from build123d import *

# Parameters (mm, degrees)
SKETCH1_R           = 57.15
SKETCH1_R_2         = 1.397
SKETCH1_R_3         = 3.175
BOSS_EXTRUDE1_DEPTH = 4.572
SKETCH2_R           = 2.75
SKETCH2_R_2         = 1.75
BOSS_EXTRUDE2_DEPTH = 2
SKETCH3_R           = 5
SKETCH3_R_2         = 1.75
BOSS_EXTRUDE3_DEPTH = 3


with BuildPart() as part:
    # Sketch1 → Boss-Extrude1 (new body)
    with BuildSketch(Plane(origin=(0, 0, 0), x_dir=(1, 0, 0), z_dir=(0, 1, 0))):
        Circle(SKETCH1_R)
        with Locations((0, 6.35)):
            Circle(SKETCH1_R_2, mode=Mode.SUBTRACT)
        with Locations((0, 25.4)):
            Circle(SKETCH1_R_3, mode=Mode.SUBTRACT)
        with Locations((0, 50.8)):
            Circle(SKETCH1_R_3, mode=Mode.SUBTRACT)
        with Locations((25.4, 0)):
            Circle(SKETCH1_R_3, mode=Mode.SUBTRACT)
        with Locations((0, -25.4)):
            Circle(SKETCH1_R_3, mode=Mode.SUBTRACT)
        with Locations((-25.4, 0)):
            Circle(SKETCH1_R_3, mode=Mode.SUBTRACT)
        with Locations((6.35, 0)):
            Circle(SKETCH1_R_2, mode=Mode.SUBTRACT)
        with Locations((0, -6.35)):
            Circle(SKETCH1_R_2, mode=Mode.SUBTRACT)
        with Locations((-6.35, 0)):
            Circle(SKETCH1_R_2, mode=Mode.SUBTRACT)
        with Locations((35.921024484, 35.921024484)):
            Circle(SKETCH1_R_3, mode=Mode.SUBTRACT)
        with Locations((50.8, 0)):
            Circle(SKETCH1_R_3, mode=Mode.SUBTRACT)
        with Locations((35.921024484, -35.921024484)):
            Circle(SKETCH1_R_3, mode=Mode.SUBTRACT)
        with Locations((0, -50.8)):
            Circle(SKETCH1_R_3, mode=Mode.SUBTRACT)
        with Locations((-35.921024484, -35.921024484)):
            Circle(SKETCH1_R_3, mode=Mode.SUBTRACT)
        with Locations((-50.8, 0)):
            Circle(SKETCH1_R_3, mode=Mode.SUBTRACT)
        with Locations((-35.921024484, 35.921024484)):
            Circle(SKETCH1_R_3, mode=Mode.SUBTRACT)
    extrude(amount=BOSS_EXTRUDE1_DEPTH)


with BuildPart() as body_2:
    # Sketch2 → Boss-Extrude2 (new body)
    with BuildSketch(Plane(origin=(0, 4.572, 0), x_dir=(1, 0, 0), z_dir=(0, 1, 0))):
        with Locations((-25.4, 0)):
            Circle(SKETCH2_R)
        with Locations((-25.4, 0)):
            Circle(SKETCH2_R_2, mode=Mode.SUBTRACT)
    extrude(amount=-BOSS_EXTRUDE2_DEPTH)

    # Sketch3 → Boss-Extrude3 (add)
    with BuildSketch(Plane(origin=(0, 4.572, 0), x_dir=(1, 0, 0), z_dir=(0, 1, 0))):
        with Locations((-25.4, 0)):
            Circle(SKETCH3_R)
        with Locations((-25.4, 0)):
            Circle(SKETCH3_R_2, mode=Mode.SUBTRACT)
    extrude(amount=BOSS_EXTRUDE3_DEPTH)


solid = body_2.part
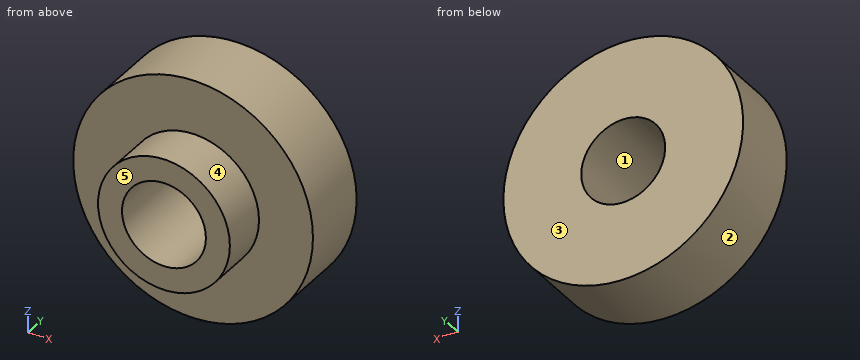
Geometry check sheet. Reference: the model listing, model coordinates, mm. Face numbers are marked on the shaded views. A direction names the side the tool comes from. Coordinates: 2 decimals unless noted, no trailing zeros. Order: outer loops, then holes, each group sorted by start corner. A loop starts at its lowest first (then second) coordinate and runs counter-clockwise, first axis right, second up. Notation, with made-up numbers: M 65.5,34 L 120.5,34 A9 ccw 120.5,41 Z; hole C 71,33 d3. An arc over 180 degrees is marked long. Use CSV: the item, a comma, the result in double quotes.
Item 1: Cross-section at D-D on z = 2. Record the cut outline in (x, y).
Returned:
outline,"M -29.98,4.57 L -27.29,4.57 L -27.29,2.57 L -23.51,2.57 L -23.51,4.57 L -20.82,4.57 L -20.82,7.57 L -29.98,7.57 Z"
Item 2: Gauge pin test, flat ends, axial feed: pin 1 Ø3 at (x, z) = (-24, -1) entering from -Y; pin 2 Ø2 at (y, z) = (6, -3.5) entering from -X; pin 3 Ø1.5 at (y, z) = (4.5, 2.5) entering from -X; pin 4 Ø1 at (y, z) = (3.5, -1) entering from -X. Record the tip position at first contact, or that the pin passes through.
Returned:
pin 1,"stops at y = 2.57"
pin 2,"stops at x = -29.73"
pin 3,"stops at x = -30.08"
pin 4,"stops at x = -28.1"
Item 3: Cross-section at B-B on x = -25.4. Record the cut outline in (y, z).
Returned:
outline,"M 2.57,-2.75 L 4.57,-2.75 L 4.57,-5 L 7.57,-5 L 7.57,-1.75 L 2.57,-1.75 Z; M 2.57,1.75 L 7.57,1.75 L 7.57,5 L 4.57,5 L 4.57,2.75 L 2.57,2.75 Z"
Item 4: Cross-section at A-A on z = 0. Record the cut outline in (x, y).
Returned:
outline,"M -30.4,4.57 L -28.15,4.57 L -28.15,2.57 L -27.15,2.57 L -27.15,7.57 L -30.4,7.57 Z; M -23.65,2.57 L -22.65,2.57 L -22.65,4.57 L -20.4,4.57 L -20.4,7.57 L -23.65,7.57 Z"
Item 5: Mould release check, pull along X, two halves, no side actions. Record for the marked faces 1, 2 and 3: pulls with the +X half, pulls with the -X half, needs draft (parallel to the pull), parting line crosses it, or undercut.
Returned:
face 1,"undercut"
face 2,"parting line crosses it"
face 3,"needs draft"
Item 6: Cross-section at C-C on y = 3.3. Record the cut outline in (x, z), then the cut area to 3 significant figures.
Returned:
outline,"C -25.4,0 d5.5; hole C -25.4,0 d3.5"
area,"14.1 mm2"
Item 7: Thickness scan on line 1 along Z through (x, y) = (-25.4, 5.7); line 2 along X through (y, z) = (3.9, 0); line 3 along X through (y, z) = (4.85, 0). Record the ranges inside material, lowest first.
Returned:
line 1,"z = -5 to -1.75, 1.75 to 5"
line 2,"x = -28.15 to -27.15, -23.65 to -22.65"
line 3,"x = -30.4 to -27.15, -23.65 to -20.4"
Item 8: Tool access check on the marked faces 4 and 5. Record the directions out of +Z, -Z, +X, -X, +Y, -Y that give a thin tool (end or side, any length) a straight path to the whole face; none if there is none.
Returned:
face 4,"-Y"
face 5,"+Z, -Z, +X, -X, -Y"
